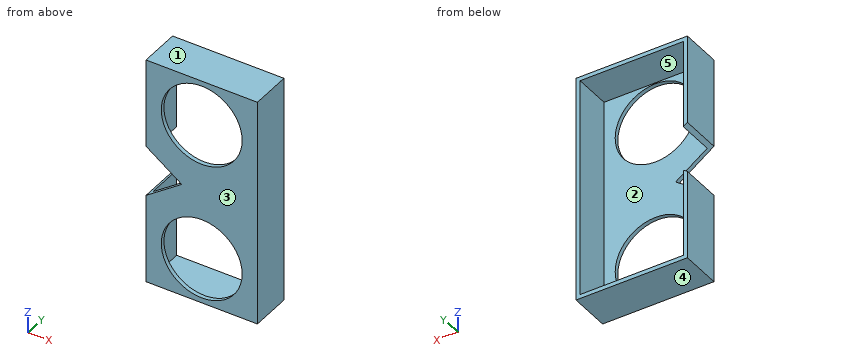
```python
from build123d import *

# Parameters (mm, degrees)
F0_W     = 68
F0_H     = 140
F1_DEPTH = 12.5
F2_T     = -2.5
F3_R     = 24.694221
F4_DEPTH = 150


with BuildPart() as f1:
    # F0 (on Front) → F1 (new body, symmetric)
    with BuildSketch(Plane.XZ):
        Rectangle(F0_W, F0_H)
    extrude(amount=F1_DEPTH, both=True)

    # F2
    f2_openings = [f1.faces().sort_by_distance(p)[0] for p in [
        (0, 12.5, 0),
    ]]
    offset(amount=F2_T, openings=f2_openings)

    # F3 (on face) → F4 (cut, symmetric)
    with BuildSketch(Plane.XZ.offset(12.5)):
        with Locations((0, 42.172134)):
            Circle(F3_R)
        with Locations((0, -42.172134)):
            Circle(F3_R)
        Polygon((-12.192623, 0), (-34, 15.491804), (-34, -15.491804), align=None)
    extrude(amount=F4_DEPTH, both=True, mode=Mode.SUBTRACT)


solid = f1.part
```
Geometry check sheet. Reference: the model listing, model coordinates, mm. Face numbers are marked on the shaded views. A direction names the side the tool comes from. Coordinates: 2 decimals unless noted, no trailing zeros. Order: outer loops, then holes, each group sorted by start corner. A loop starts at its lowest first (then second) coordinate and runs counter-clockwise, first axis right, second up. Notation, with made-up numbers: (-3, 4.5) - (46, 4.5) arc R28 cw to (46, 27.5) - close; hole circle Ø9 at (87.25, 25.25). An arc over 180 degrees is marked (long way). Answer as a JSON object with one key per item and string values. Group by question number.
Item 1: Tool access check on the marked faces 4 and 5. Record the directions out of +Z, -Z, +X, -X, +Y, -Y that give a thin tool (end or side, any length) a straight path to the whole face; none if there is none.
Item 2: Scan lines: probe 1 along Z at (x, y) = (0, -11.5); probe 2 along X at (y, z) = (3.75, 42.5); probe 3 along Z at (x, y) = (-11, -6.5). Record each from-to range of solid material in increasing order.
Item 3: Sectioned sample at A-A, the plane x = 0. Record the cut outline in (y, z), and give its area (3 significant figures).
Item 4: Depth check by flat-ended pin: pin 1 Ø5 at (y, z) = (-2, 0) entering from -X; pin 2 Ø4 at (x, z) = (-5.5, 10) entering from +Y. Enter the tip coordinate at first touch or a pass-through.
Item 5: Draft check along Z on the marked faces 1, 2 and 3. Enter one of: +Z half, -Z half, draft (parallel to the pull), parting line (faces both ways), or undercut.
Item 6: Sectioned sample at B-B, the plane z = -40. Record the cut outline in (x, y).
Item 7: Sectioned sample at C-C, the plane y = 3.75. Record the cut outline in (x, z), and give its area (3 significant figures).
Item 8: Sectioned sample at D-D, the plane x = -28. Record the cut outline in (y, z).
Resolved:
{
 "1": {"face 4": "-Z, +X, -X, +Y, -Y", "face 5": "+Y"},
 "2": {"probe 1": "-70 to -66.87, -17.48 to 17.48, 66.87 to 70", "probe 2": "-34 to -31.5, 31.5 to 34", "probe 3": "-70 to -67.5, 67.5 to 70"},
 "3": {"outline": "(-12.5, -70) - (12.5, -70) - (12.5, -67.5) - (-10, -67.5) - (-10, -66.87) - (-12.5, -66.87) - close; (-12.5, -17.48) - (-10, -17.48) - (-10, 17.48) - (-12.5, 17.48) - close; (-12.5, 66.87) - (-10, 66.87) - (-10, 67.5) - (12.5, 67.5) - (12.5, 70) - (-12.5, 70) - close", "area": "216 mm^2"},
 "4": {"pin 1": "x = 31.5", "pin 2": "y = -10"},
 "5": {"face 1": "+Z half", "face 2": "undercut", "face 3": "draft"},
 "6": {"outline": "(-34, -12.5) - (-24.6, -12.5) - (-24.6, -10) - (-31.5, -10) - (-31.5, 12.5) - (-34, 12.5) - close; (24.6, -12.5) - (34, -12.5) - (34, 12.5) - (31.5, 12.5) - (31.5, -10) - (24.6, -10) - close"},
 "7": {"outline": "(-34, -70) - (34, -70) - (34, 70) - (-34, 70) - (-34, 15.49) - (-31.5, 13.72) - (-31.5, 67.5) - (31.5, 67.5) - (31.5, -67.5) - (-31.5, -67.5) - (-31.5, -13.72) - (-34, -15.49) - close", "area": "942 mm^2"},
 "8": {"outline": "(-12.5, -70) - (12.5, -70) - (12.5, -67.5) - (-10, -67.5) - (-10, -11.23) - (-12.5, -11.23) - close; (-12.5, 11.23) - (-10, 11.23) - (-10, 67.5) - (12.5, 67.5) - (12.5, 70) - (-12.5, 70) - close"}
}
